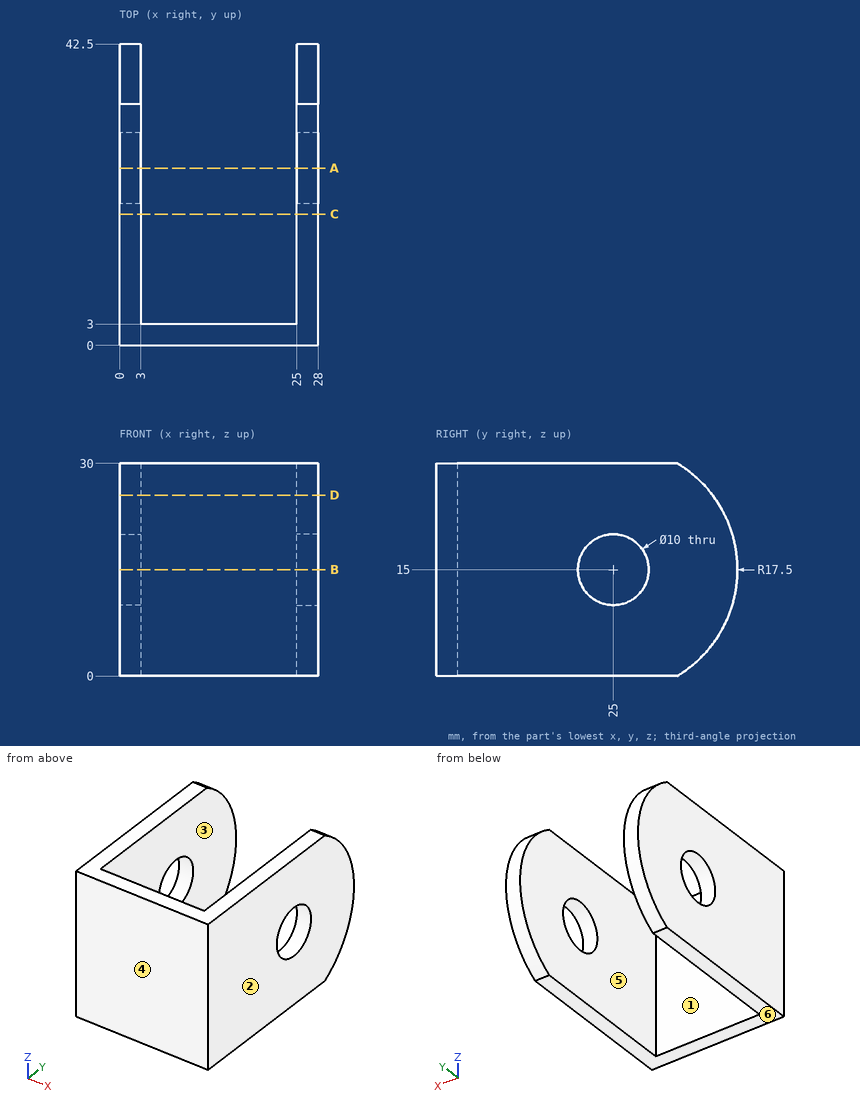
For this review, use the dimensioned drawing (mm, ordinates from the lowest corner) and the shaded views. A direction names the side the tool comes from. Round coordinates to 2 decimals unless told otherwise and drop trailing zeros. Write each loop counter-clockwise with the first axis right and the second up, starting at its lowest first coordinate (ties: lowest second). Pieces come first, ordered by that corner, then holes. Notation, with made-up numbers: (35.5, 20) - (42.5, 20) arc R22 cw to (42.5, 35) - close; hole circle Ø9 at (69.25, 20.5). An arc over 180 degrees is marked (long way). One line per item, written item: value. Start each with the question number.
1. Consider section A-A on y = 25. Write out the cut boundary in (x, z), and give its area (3 significant figures).
2. To check wall thickness, follow L1, parallel to X at y = 18.5, z = 10; L2, parallel to Z at x = 25.6, y = 25; L3, parallel to Y at x = 26.6, z = 15. State the ranges of each line that lie inside material, in increasing order. Write a range as from..to.
3. Consider section C-C on y = 18.5. Write out the cut boundary in (x, z), and give its area (3 significant figures).
4. Machinability: for the marked faces 5 and 6, which of the approach directions +Z, -Z, +X, -X, +Y, -Y give a long, thin tool a straight path to every point of the face, cutting with its end or side? Answer none if there is none.
5. Consider section D-D on z = 25.5. Write out the cut boundary in (x, y).
6. The part is to be moulded in two halves that separate along X. For the marked faces 1, 2, 3 and 4, say which applies: released by +X, released by -X, zero draft, split by the parting line, or undercut.
7. Clearance check with flat-ended pins moving along their axes: P1, Ø6, axis at y = 25, z = 15, coming from the +X side; P2, Ø3, axis at x = 17.5, z = 12, coming from the +Y side. State where each tip first meets the part, or that it passes through.
8. Consider section B-B on z = 15. Write out the cut boundary in (x, y).
Checks:
1. outline: (0, 0) - (3, 0) - (3, 10) - (0, 10) - close; (0, 20) - (3, 20) - (3, 30) - (0, 30) - close; (25, 0) - (28, 0) - (28, 10) - (25, 10) - close; (25, 20) - (28, 20) - (28, 30) - (25, 30) - close
1. area: 120 mm^2
2. L1: x = 0..3, 25..28
2. L2: z = 0..10, 20..30
2. L3: y = 0..20, 30..42.5
3. outline: (0, 0) - (3, 0) - (3, 30) - (0, 30) - close; (25, 0) - (28, 0) - (28, 30) - (25, 30) - close
3. area: 180 mm^2
4. face 5: +Z, -Z, +Y
4. face 6: -Z, +X, -X, +Y, -Y
5. outline: (0, 0) - (28, 0) - (28, 39) - (25, 39) - (25, 3) - (3, 3) - (3, 39) - (0, 39) - close
6. face 1: undercut
6. face 2: released by +X
6. face 3: undercut
6. face 4: zero draft
7. P1: passes through
7. P2: stops at y = 3
8. outline: (0, 0) - (28, 0) - (28, 20) - (25, 20) - (25, 3) - (3, 3) - (3, 20) - (0, 20) - close; (0, 30) - (3, 30) - (3, 42.5) - (0, 42.5) - close; (25, 30) - (28, 30) - (28, 42.5) - (25, 42.5) - close
